The model under review builds one solid part; all positions refer to its coordinate system, in mm. Face numbers are marked on the shaded views. A direction names the side the tool comes from. Round coordinates to 2 decimals unless told otherwise and drop trailing zeros. Loops run counter-clockwise (first coordinate to the right, second up) from the corner with the lowest first, then second, coordinate; pieces in that order, holes last. Notation, with made-up numbers: (26, -11) -> (58, -11) arc R14 cw to (58, 5) -> close; hole circle Ø11 at (-10, 58.5). An arc over 180 degrees is marked (long way). Use a Markdown table: item, result. Add a question column.
1) Mouldability with a two-part tool opening along X and no side actions: class the marked faces 6, 7 and 8 as released by +X, released by -X, zero draft, split by the parting line, or undercut.
2) Consider section D-D on z = 9.5. Give the boundary of the cut face in (x, y), plus the area to 3 significant figures.
3) For the marked faces 1, 2, 3, 4 and 5, list the 3-axis set-ups (+Z, -Z, +X, -X, +Y, -Y) from which the entire face can be reached by the end or side of a thin tool; tool diameter is ignored.
4) Insertion check: pin 1 (12 mm diameter, centred on y = 6.5, z = 10, fed in from -X); pin 2 (12 mm diameter, centred on x = -43, z = -3, fed in from +Y); pin 3 (5.5 mm diameter, centred on x = 35.5, z = 5, fed in from -Y). Each pin has a flat end and moves straight along its axis. Give the tip position at first contact, or say it passes through.
5) Consider section A-A on z = -4.5. Give the boundary of the cut face in (x, y).
6) Consider section C-C on y = -14. Give the boundary of the cut face in (x, z).
7) Consider section B-B on x = -42.5. Give the boundary of the cut face in (y, z).
8) Wall thickness on probe 1 along Z at (x, y) = (-42.5, -14.5); probe 2 along X at (y, z) = (-15.3, -4.5); probe 3 along Z at (x, y) = (-42, -14): over which ranges is each line inside the solid? List them lowest first.
from build123d import *

# Parameters (mm, degrees)
BOSS_EXTRUDE1_DEPTH     = 30
SKETCH2_W               = 50
SKETCH2_H               = 20
CUT_EXTRUDE1_DEPTH      = 30
CHAMFER1_SIZE           = 2
SKETCH3_R               = 2.1
CUT_EXTRUDE2_DEPTH      = 30
SKETCH6_W               = 5
SKETCH6_H               = 30
BOSS_EXTRUDE2_DEPTH     = 5
SKETCH7_W               = 126.18944296
SKETCH7_H               = 49.64624499
CUT_EXTRUDE3_DEPTH      = 15
SKETCH8_W               = 20
SKETCH8_H               = 15
BOSS_EXTRUDE3_DEPTH     = 5
SKETCH9_W               = 71
SKETCH9_H               = 15
BOSS_EXTRUDE4_DEPTH     = 5
SKETCH10_W              = 15
SKETCH10_H              = 20
SKETCH10_H_2            = 5
CUT_EXTRUDE4_DEPTH      = 38
CUT_EXTRUDE4_DEPTH_BACK = 27
SKETCH11_R              = 2.1
CUT_EXTRUDE5_DEPTH      = 27
SKETCH12_R              = 2.1
BOSS_EXTRUDE5_DEPTH     = 5
SKETCH13_R              = 2.1
CUT_EXTRUDE6_DEPTH      = 5
SKETCH14_W              = 5
SKETCH14_H              = 15
CUT_EXTRUDE7_DEPTH      = 10
SKETCH15_W              = 5
SKETCH15_H              = 15
CUT_EXTRUDE8_DEPTH      = 10
SKETCH16_W              = 10
SKETCH16_H              = 25
BOSS_EXTRUDE6_DEPTH     = 5
SKETCH17_R              = 2.1
CUT_EXTRUDE9_DEPTH      = 30
SKETCH18_W              = 10
SKETCH18_H              = 5
BOSS_EXTRUDE7_DEPTH     = 5
CHAMFER3_SIZE           = 1
CHAMFER4_SIZE           = 1


with BuildPart() as part:
    # Sketch1 → Boss-Extrude1 (new body)
    with BuildSketch(Plane.XY):
        Polygon((-57.5, -17.5), (-37.5, -17.5), (-32.5, -17.5), (-32.5, 12.5), (32.5, 12.5), (32.5, -17.5), (37.5, -17.5), (57.5, -17.5), (57.5, -12.5), (37.5, -12.5), (37.5, 17.5), (-37.5, 17.5), (-37.5, -12.5), (-57.5, -12.5), align=None)
    extrude(amount=BOSS_EXTRUDE1_DEPTH)

    # Sketch2 → Cut-Extrude1 (cut)
    with BuildSketch(Plane(origin=(0, 17.5, 0), x_dir=(1, 0, 0), z_dir=(0, 1, 0))):
        with Locations((0, -15)):
            Rectangle(SKETCH2_W, SKETCH2_H)
    extrude(amount=-CUT_EXTRUDE1_DEPTH, mode=Mode.SUBTRACT)

    # Chamfer1
    chamfer1_edges = [part.edges().sort_by_distance(p)[0] for p in [
        (-37.5, 17.5, 15),
        (37.5, 17.5, 15),
    ]]
    chamfer(chamfer1_edges, length=CHAMFER1_SIZE)

    # Sketch3 → Cut-Extrude2 (cut)
    with BuildSketch(Plane(origin=(0, -12.5, 0), x_dir=(1, 0, 0), z_dir=(0, 1, 0))):
        with Locations((-47.5, -15)):
            Circle(SKETCH3_R)
        with Locations((47.5, -15)):
            Circle(SKETCH3_R)
    extrude(amount=-CUT_EXTRUDE2_DEPTH, mode=Mode.SUBTRACT)

    # Sketch6 → Boss-Extrude2 (add)
    with BuildSketch(Plane(origin=(0, 17.5, 0), x_dir=(1, 0, 0), z_dir=(0, 1, 0))):
        with Locations((0, -15)):
            Rectangle(SKETCH6_W, SKETCH6_H)
    extrude(amount=-BOSS_EXTRUDE2_DEPTH)

    # Sketch7 → Cut-Extrude3 (cut)
    with BuildSketch(Plane.XY.offset(30)):
        Rectangle(SKETCH7_W, SKETCH7_H)
    extrude(amount=-CUT_EXTRUDE3_DEPTH, mode=Mode.SUBTRACT)

    # Sketch8 → Boss-Extrude3 (add, through all)
    with BuildSketch(Plane(origin=(0, -12.5, 0), x_dir=(1, 0, 0), z_dir=(0, 1, 0))):
        with Locations((-47.5, -7.5)):
            Rectangle(SKETCH8_W, SKETCH8_H)
    extrude(amount=-BOSS_EXTRUDE3_DEPTH)

    # Sketch9 → Boss-Extrude4 (add)
    with BuildSketch(Plane(origin=(0, 17.5, 0), x_dir=(1, 0, 0), z_dir=(0, 1, 0))):
        with Locations((0, -7.5)):
            Rectangle(SKETCH9_W, SKETCH9_H)
    extrude(amount=-BOSS_EXTRUDE4_DEPTH)

    # Sketch10 → Cut-Extrude4 (cut, two sides)
    with BuildSketch(Plane(origin=(37.5, 0, 0), x_dir=(0, 0, -1), z_dir=(1, 0, 0))) as cut_extrude4_sk:
        with Locations((-7.5, -2.5)):
            Rectangle(SKETCH10_W, SKETCH10_H)
        with Locations((-7.5, -15)):
            Rectangle(SKETCH10_W, SKETCH10_H_2)
    extrude(amount=CUT_EXTRUDE4_DEPTH, mode=Mode.SUBTRACT)
    extrude(cut_extrude4_sk.sketch, amount=-CUT_EXTRUDE4_DEPTH_BACK, mode=Mode.SUBTRACT)

    # Sketch11 → Cut-Extrude5 (cut)
    with BuildSketch(Plane(origin=(0, -12.5, 0), x_dir=(1, 0, 0), z_dir=(0, 1, 0))):
        with Locations((-47.5, -7.5)):
            Circle(SKETCH11_R)
    extrude(amount=-CUT_EXTRUDE5_DEPTH, mode=Mode.SUBTRACT)

    # Sketch12 → Boss-Extrude5 (add)
    with BuildSketch(Plane(origin=(0, -17.5, 0), x_dir=(-1, 0, 0), z_dir=(0, -1, 0))):
        with Locations((47.5, -7.5)):
            Circle(SKETCH12_R)
    extrude(amount=-BOSS_EXTRUDE5_DEPTH)

    # Sketch13 → Cut-Extrude6 (cut)
    with BuildSketch(Plane(origin=(0, -17.5, 0), x_dir=(-1, 0, 0), z_dir=(0, -1, 0))):
        with Locations((42.5, -11)):
            Circle(SKETCH13_R)
        with Locations((42.5, -4)):
            Circle(SKETCH13_R)
    extrude(amount=-CUT_EXTRUDE6_DEPTH, mode=Mode.SUBTRACT)

    # Sketch14 → Cut-Extrude7 (cut)
    with BuildSketch(Plane(origin=(0, -17.5, 0), x_dir=(-1, 0, 0), z_dir=(0, -1, 0))):
        with Locations((55, -7.5)):
            Rectangle(SKETCH14_W, SKETCH14_H)
    extrude(amount=-CUT_EXTRUDE7_DEPTH, mode=Mode.SUBTRACT)

    # Sketch15 → Cut-Extrude8 (cut)
    with BuildSketch(Plane(origin=(0, -12.5, 0), x_dir=(1, 0, 0), z_dir=(0, 1, 0))):
        with Locations((-50, -7.5)):
            Rectangle(SKETCH15_W, SKETCH15_H)
    extrude(amount=-CUT_EXTRUDE8_DEPTH, mode=Mode.SUBTRACT)

    # Sketch16 → Boss-Extrude6 (add, through all)
    with BuildSketch(Plane(origin=(0, -12.5, 0), x_dir=(1, 0, 0), z_dir=(0, 1, 0))):
        with Locations((-42.5, -2.5)):
            Rectangle(SKETCH16_W, SKETCH16_H)
    extrude(amount=-BOSS_EXTRUDE6_DEPTH)

    # Sketch17 → Cut-Extrude9 (cut)
    with BuildSketch(Plane(origin=(0, -12.5, 0), x_dir=(1, 0, 0), z_dir=(0, 1, 0))):
        with Locations((-42.5, 4.5)):
            Circle(SKETCH17_R)
        with Locations((-42.5, -9.5)):
            Circle(SKETCH17_R)
    extrude(amount=-CUT_EXTRUDE9_DEPTH, mode=Mode.SUBTRACT)

    # Sketch18 → Boss-Extrude7 (add)
    with BuildSketch(Plane(origin=(-37.5, 0, 0), x_dir=(0, 0, -1), z_dir=(1, 0, 0))):
        with Locations((5, -15)):
            Rectangle(SKETCH18_W, SKETCH18_H)
    extrude(amount=BOSS_EXTRUDE7_DEPTH)

    # Chamfer3
    chamfer3_edges = [part.edges().sort_by_distance(p)[0] for p in [
        (-47.5, -15, 15),
        (-47.5, -15, -10),
    ]]
    chamfer(chamfer3_edges, length=CHAMFER3_SIZE)

    # Chamfer4
    chamfer4_edges = [part.edges().sort_by_distance(p)[0] for p in [
        (-32.5, -15, -10),
    ]]
    chamfer(chamfer4_edges, length=CHAMFER4_SIZE)


solid = part.part
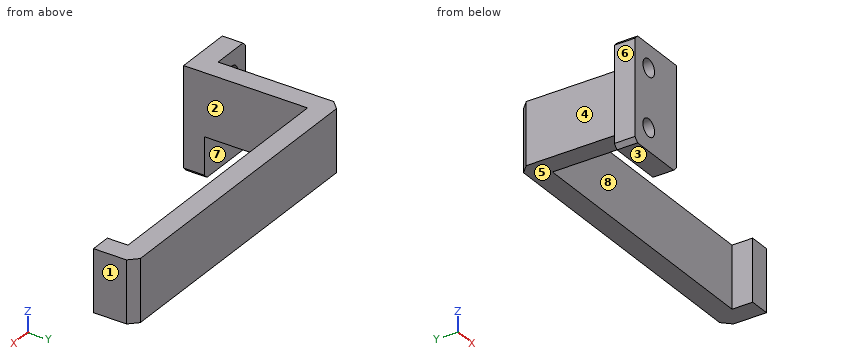
Result set:
| question | item | result |
|---|---|---|
| 1 | face 6 | released by -X |
| 1 | face 7 | zero draft |
| 1 | face 8 | undercut |
| 2 | outline | (-47.5, -17.5) -> (-44.6, -17.5) -> (-44.6, -12.5) -> (-47.5, -12.5) -> close; (-40.4, -17.5) -> (-32.5, -17.5) -> (-32.5, 12.5) -> (32.5, 12.5) -> (32.5, 7.5) -> (37.5, 7.5) -> (37.5, 15.5) -> (35.5, 17.5) -> (-35.5, 17.5) -> (-37.5, 15.5) -> (-37.5, -12.5) -> (-40.4, -12.5) -> close |
| 2 | area | 575 mm2 |
| 3 | face 1 | +Z, -Z, +X, +Y, -Y |
| 3 | face 2 | +Z, -Z, -Y |
| 3 | face 3 | -Z, +X, -X, +Y, -Y |
| 3 | face 4 | +Z, -Z, -X, +Y |
| 3 | face 5 | -Z, +X, -X, +Y |
| 4 | pin 1 | x = -37.5 |
| 4 | pin 2 | y = -12.5 |
| 4 | pin 3 | y = 7.5 |
| 5 | outline | (-47.5, -17.5) -> (-44.6, -17.5) -> (-44.6, -12.5) -> (-47.5, -12.5) -> close; (-40.4, -17.5) -> (-32.5, -17.5) -> (-32.5, -12.5) -> (-40.4, -12.5) -> close |
| 6 | outline | (-47.5, -9) -> (-46.5, -10) -> (-33.5, -10) -> (-32.5, -9) -> (-32.5, 15) -> (-46.5, 15) -> (-47.5, 14) -> close; hole circle Ø4.2 at (-42.5, -4.5); hole circle Ø4.2 at (-42.5, 9.5) |
| 7 | outline | (-17.5, -10) -> (-12.5, -10) -> (-12.5, -6.6) -> (-17.5, -6.6) -> close; (-17.5, -2.4) -> (-12.5, -2.4) -> (-12.5, 7.4) -> (-17.5, 7.4) -> close; (-17.5, 11.6) -> (-12.5, 11.6) -> (-12.5, 15) -> (-17.5, 15) -> close |
| 8 | probe 1 | -10 to -6.6, -2.4 to 7.4, 11.6 to 15 |
| 8 | probe 2 | -47.5 to -44.6, -40.4 to -32.5 |
| 8 | probe 3 | -10 to -6.54, -2.46 to 7.46, 11.54 to 15 |
